from build123d import *

# Parameters (mm, degrees)
SKETCH001_W  = 230
SKETCH001_H  = 8
PAD001_DEPTH = 4
CHAMFER_SIZE = 7.99
FILLET_R     = 7.99


with BuildPart() as part:
    # Sketch001 → Pad001 (new body, symmetric)
    with BuildSketch(Plane.XZ):
        Rectangle(SKETCH001_W, SKETCH001_H)
    extrude(amount=PAD001_DEPTH, both=True)

    # Chamfer
    chamfer_edges = [part.edges().sort_by_distance(p)[0] for p in [
        (115, 0, 4),
        (-115, 0, 4),
    ]]
    chamfer(chamfer_edges, length=CHAMFER_SIZE)

    # Fillet
    fillet_edges = [part.edges().sort_by_distance(p)[0] for p in [
        (0, 4, 4),
    ]]
    fillet(fillet_edges, radius=FILLET_R)


solid = part.part
Design review of the part built by this model. Coordinates are the model's own, in mm. Coordinates: 2 decimals unless noted, no trailing zeros. Write each loop counter-clockwise with the first axis right and the second up, starting at its lowest first coordinate (ties: lowest second). Pieces come first, ordered by that corner, then holes. Notation, with made-up numbers: (53, 38) -> (80, 38) arc R10 ccw to (80, 48) -> close; hole circle Ø9 at (-28, 80.25). An arc over 180 degrees is marked (long way). Write each question's results on one line, items separated by ' | '. Start each with the question number.
(1) For line 1 along Z through (x, y) = (23, -3.5); line 2 along Z through (x, y) = (-32, -1.5); line 3 along Y through (x, z) = (-57.5, 0.75), list the stretches that pass through material, from the lowest coordinate up. Write a range as from..to.
(2) Clearance check with a flat-ended pin moving along its axis: P1, Ø3, axis at y = 1, z = 0, coming from the -X side. State where the tip first meets the part, or that it passes through.
(3) The part is to be moulded in two halves that separate along Z. For faces 1 (the face through (-2, -4, 0)), 2 (the face through (-2, 0, -4)), 3 (the face through (111.84, -0.94, -0.83)), say which applies: pulls with the +Z half, pulls with the -Z half, needs draft (parallel to the pull), parting line crosses it, or undercut.
(4) Take a section at C-C on z = 2. Write out the cut boundary in (x, y).
Results found:
1) line 1: z = -4..3.98 | line 2: z = -4..3.6 | line 3: y = -4..2.44
2) P1: stops at x = -112.51
3) face 1: needs draft | face 2: pulls with the -Z half | face 3: pulls with the +Z half
4) outline: (-109.01, -4) -> (109.01, -4) -> (109.01, 1.3) -> (-109.01, 1.3) -> close
